Could you check a few things on this drawing? It's one solid part, dimensions in mm from its lowest x, y, z. A direction names the side the tool comes from. Coordinates: 2 decimals unless noted, no trailing zeros. Loops run counter-clockwise (first coordinate to the right, second up) from the corner with the lowest first, then second, coordinate; pieces in that order, holes last. Notation, with made-up numbers: (44, -19.5) -> (68, -19.5) arc R18 cw to (68, -4.5) -> close; hole circle Ø1 at (-29, 86.5). An arc over 180 degrees is marked (long way). One line per question, with ' | ' between items.
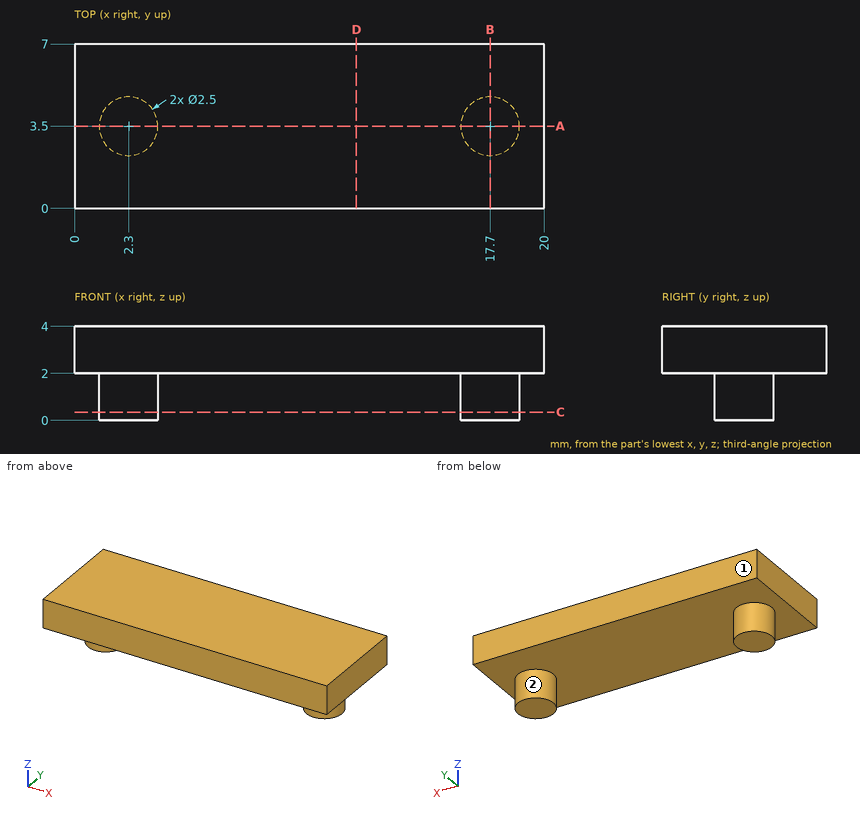
1) If we section it at B-B on x = 17.7: Please give me the cut outline in (y, z), and give its area (3 significant figures).
Data:
outline: (0, 2) -> (2.25, 2) -> (2.25, 0) -> (4.75, 0) -> (4.75, 2) -> (7, 2) -> (7, 4) -> (0, 4) -> close | area: 19.0 mm²
2) On a 3-axis mill with a long thin cutter (end or side, diameter ignored), from which of +Z, -Z, +X, -X, +Y, -Y can I reach the whole of each face in a straight line? I mean the marked faces 1 and 2. Say none if no direction works.
Data:
face 1: +Z, -Z, +X, -X, +Y | face 2: -Z
3) If we section it at A-A on y = 3.5: Please give me the cut outline in (x, z).
Data:
outline: (0, 2) -> (1.05, 2) -> (1.05, 0) -> (3.55, 0) -> (3.55, 2) -> (16.45, 2) -> (16.45, 0) -> (18.95, 0) -> (18.95, 2) -> (20, 2) -> (20, 4) -> (0, 4) -> close
4) If we section it at D-D on x = 12: Please give me the cut outline in (y, z), and give its area (3 significant figures).
Data:
outline: (0, 2) -> (7, 2) -> (7, 4) -> (0, 4) -> close | area: 14.0 mm²
5) If we section it at C-C on z = 0.35: Please give me the cut outline in (x, y).
Data:
outline: circle Ø2.5 at (2.3, 3.5); circle Ø2.5 at (17.7, 3.5)
6) I need wall thicknesses on line 1 along Z through (x, y) = (2, 1.5); line 2 along X through (y, z) = (3.25, 0.35); line 3 along Y through (x, z) = (1.5, 1.55). Which ranges of each line are inside material? Lowest first, please. Write a range as from..to.
Data:
line 1: 2..4 | line 2: 1.08..3.52, 16.48..18.92 | line 3: 2.54..4.46
7) I'm going to push a flat-ended pin straight in: pin 1 Ø1.5 at (y, z) = (2.5, 0.5) entering from +X. Where does the tip first touch, or does it pass through?
Data:
pin 1: x = 18.92
